```python
from build123d import *

# Parameters (mm, degrees)
BOSS_EXTRUDE1_DEPTH          = 5.08
F_3_8_0_375_DIAMETER_HOLE1_D = 9.525
F_3_8_0_375_DIAMETER_HOLE2_D = 9.525


with BuildPart() as part:
    # Sketch1 → Boss-Extrude1 (new body)
    with BuildSketch(Plane(origin=(0, 0, 0), x_dir=(1, 0, 0), z_dir=(0, 1, 0))):
        with BuildLine():
            Line((186.706216966, -778.102360844), (-171.269771153, -778.102360844))
            add(Edge.make_bspline(
                [(-171.269771153, -778.102360844), (-159.707774454, -836.134775395), (-146.81892484, -893.9188082), (-132.611103769, -951.360767835), (-118.403260068, -1008.802818957), (-102.873342202, -1065.933903144), (-86.045569786, -1122.663773012), (-74.990089761, -1159.934062127), (-63.371281317, -1197.041907081), (-51.194215445, -1233.960969312), (-45.100567198, -1252.436009294), (-38.866841431, -1270.865430421), (-32.494599583, -1289.246240662), (-26.120797202, -1307.631552278), (-20.652525047, -1326.386680917), (-12.917829919, -1344.242199148)],
                knots=[0, 0, 0, 0, 0.177518923, 0.177518923, 0.177518923, 0.355038121, 0.355038121, 0.355038121, 0.471646972, 0.471646972, 0.471646972, 0.529995372, 0.529995372, 0.529995372, 0.588358391, 0.588358391, 0.588358391, 0.588358391], degree=3))
            ThreePointArc((-12.917829919, -1344.242199148), (7.718222897, -1357.79203399), (28.354275723, -1344.242199164))
            add(Edge.make_bspline(
                [(28.354275723, -1344.242199164), (38.120725658, -1321.696381858), (44.939237661, -1298.079369173), (60.823654171, -1251.671639351), (68.544496879, -1228.393431097), (91.029194373, -1158.368706478), (105.122355407, -1111.420274649), (144.723795491, -969.782644477), (167.537266257, -874.315888923), (186.706216966, -778.102360844)],
                knots=[0, 0, 0, 0, 0.125, 0.125, 0.25, 0.25, 0.5, 0.5, 1, 1, 1, 1], degree=3))
        make_face()
    extrude(amount=BOSS_EXTRUDE1_DEPTH)

    # 3/8 (0.375) Diameter Hole1 (through all)
    with Locations(Plane(origin=(0, 5.08, 0), x_dir=(1, 0, 0), z_dir=(0, 1, 0))):
        with Locations((7.718222897, -1326.04203399), (7.718222897, -1300.64203399)):
            Hole(F_3_8_0_375_DIAMETER_HOLE1_D / 2)

    # 3/8 (0.375) Diameter Hole2 (through all)
    with Locations(Plane(origin=(0, 5.08, 0), x_dir=(1, 0, 0), z_dir=(0, 1, 0))):
        with Locations((-49.431777094, -970.44203399), (-49.431777094, -1008.54203399), (64.868222906, -970.44203399), (64.868222906, -1008.54203399), (-11.331777094, -1205.39203399), (26.768222906, -1205.39203399)):
            Hole(F_3_8_0_375_DIAMETER_HOLE2_D / 2)


solid = part.part
```
Geometry check sheet. Reference: the model listing, model coordinates, mm. Coordinates: 2 decimals unless noted, no trailing zeros. Answer as a JSON object with one key per item and string values. Group by question number.
Item 1: Sectioned sample at A-A, the plane y = 1.3. Give the number of separate pieces and of enclosed holes in the cut face, and give its area (3 significant figures).
Item 2: Scan lines: probe 1 along X at (y, z) = (2.45, 1207); probe 2 along Z at (x, y) = (5, 1.4); probe 3 along X at (y, z) = (2.55, 1012). Record each from-to range of solid material in increasing order.
Item 3: Depth check by flat-ended pin: pin 1 Ø7.5 at (x, z) = (26.77, 1205.39) entering from +Y; pin 2 Ø11 at (x, z) = (-11.33, 1205.39) entering from -Y. Enter the tip coordinate at first touch or a pass-through.
Resolved:
{
 "1": {"separate pieces": "1", "enclosed holes": "8", "area": "122,000 mm^2"},
 "2": {"probe 1": "-59.98 to -15.81, -6.85 to 22.29, 31.25 to 75.41", "probe 2": "778.1 to 1296.73, 1304.55 to 1322.13, 1329.95 to 1357.63", "probe 3": "-117.09 to -52.71, -46.16 to 61.59, 68.14 to 132.53"},
 "3": {"pin 1": "through", "pin 2": "y = 0"}
}
